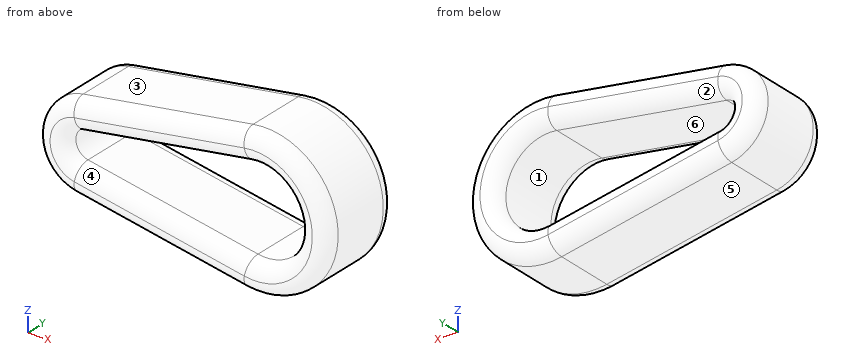
from build123d import *

# Parameters (mm, degrees)
F1_DEPTH      = 15
F1_DEPTH_BACK = 15
F2_R          = 4.99999


# Not quite as in the source:
# - a fillet or chamfer is up to 0.001 mm smaller than in the source, because OpenCascade refuses the exact size


with BuildPart() as f1:
    # F0 (on Front) → F1 (new body, two sides)
    with BuildSketch(Plane.XZ) as f1_sk:
        with BuildLine():
            Line((-2.5, -14.7901994577), (55.8333333333, -24.6503324296))
            ThreePointArc((55.8333333333, -24.6503324296), (85, 0), (55.8333333333, 24.6503324296))
            Line((55.8333333333, 24.6503324296), (-2.5, 14.7901994577))
            ThreePointArc((-2.5, 14.7901994577), (-15, 0), (-2.5, -14.7901994577))
        make_face()
        with BuildLine():
            ThreePointArc((-0.8333333333, -4.9300664859), (-5, 0), (-0.8333333333, 4.9300664859))
            Line((-0.8333333333, 4.9300664859), (57.5, 14.7901994577))
            ThreePointArc((57.5, 14.7901994577), (75, 0), (57.5, -14.7901994577))
            Line((57.5, -14.7901994577), (-0.8333333333, -4.9300664859))
        make_face(mode=Mode.SUBTRACT)
    extrude(amount=F1_DEPTH)
    extrude(f1_sk.sketch, amount=-F1_DEPTH_BACK)

    # F2 (radius 5 in the source; OpenCascade refuses exactly that, so slightly less here)
    f2_edges = [f1.edges().sort_by_distance(p)[0] for p in [
        (28.333333, -15, 9.860133),
        (26.666667, -15, 19.720266),
        (26.666667, 15, 19.720266),
        (28.333333, 15, 9.860133),
    ]]
    fillet(f2_edges, radius=F2_R)


solid = f1.part
Geometry check sheet. Reference: the model listing, model coordinates, mm. Face numbers are marked on the shaded views. A direction names the side the tool comes from. Round coordinates to 2 decimals unless told otherwise and drop trailing zeros. Write each loop counter-clockwise with the first axis right and the second up, starting at its lowest first coordinate (ties: lowest second). Pieces come first, ordered by that corner, then holes.
Item 1: Go/stop test with flat-tipped pins: pin 1 Ø6 at (x, y) = (50.5, -10.5) entering from +Z; pin 2 Ø3 at (x, z) = (42.5, 13) entering from +Y; pin 3 Ø5 at (x, y) = (4.5, 6) entering from -Z; pin 4 Ø1 at (x, z) = (3.5, 4) entering from -Y. Record where each tip stops, or that it passes through.
Determined:
pin 1: stops at z = 24.25
pin 2: stops at y = 14.17
pin 3: stops at z = -16.4
pin 4: passes through
Item 2: Mould release check, pull along X, two halves, no side actions. Record for the marked faces 1, 2 and 3: +X half, -X half, draft (parallel to the pull), parting line (faces both ways), or undercut.
Determined:
face 1: undercut
face 2: undercut
face 3: -X half
Item 3: Section check C-C (y = 13.25). Record the boundary of the cut face in (x, z).
Determined:
outline: (-2.3, -13.61) - (56.03, -23.47) arc R23.8 ccw (long way) to (56.03, 23.47) - (-2.3, 13.61) arc R13.8 ccw to start; hole (-1.03, -6.11) - (57.3, -15.97) arc R16.2 ccw (long way) to (57.3, 15.97) - (-1.03, 6.11) arc R6.2 ccw to start
Item 4: Section check B-B (y = -0.75). Record the boundary of the cut face in (x, z).
Determined:
outline: (-2.5, -14.79) - (55.83, -24.65) arc R25 ccw (long way) to (55.83, 24.65) - (-2.5, 14.79) arc R15 ccw to start; hole (-0.83, -4.93) - (57.5, -14.79) arc R15 ccw (long way) to (57.5, 14.79) - (-0.83, 4.93) arc R5 ccw to start
Item 5: Access from +Z, -Z, +X, -X, +Y, -Y to the whole of each face (thin tool, end or side, straight path). Record for the marked faces 4, 5 and 6.
Determined:
face 4: -Y
face 5: -Z, -X, +Y, -Y
face 6: +Y, -Y
Item 6: Material ranges on line 1 along Z through (x, y) = (60, 2); line 2 along Y through (x, z) = (77.5, 9); line 3 along Z through (x, y) = (71.5, -2), recorded low to high.
Determined:
line 1: z = -25 to -15, 15 to 25
line 2: y = -14.99 to 14.99
line 3: z = -22.2 to -9.63, 9.63 to 22.2
